Read the model definition and answer for the solid it produces. Units are mm, in the model's axes. A direction names the side the tool comes from. Round coordinates to 2 decimals unless told otherwise and drop trailing zeros. Write each loop counter-clockwise with the first axis right and the second up, starting at its lowest first coordinate (ties: lowest second). Pieces come first, ordered by that corner, then holes. Notation, with made-up numbers: (26.5, 6) - (48.5, 6) arc R14 ccw to (48.5, 24) - close; hole circle Ø3 at (83.25, 38). An arc over 180 degrees is marked (long way). One line per item, written item: value. Start each with the question number.
(1) A cutting plane is placed at B-B, the plane x = 0. Determine the outline of the cut face in (y, z).
(2) For faces 4 (the face through (39, 10.483, 9)), 5 (the face through (-1.172, 8.923, 17.902)), 6 (the face through (-39, 10.483, 9)), determine the directions among +Z, -Z, +X, -X, +Y, -Y from which every point of the face is accessible in a straight line to the end or side of a thin tool.
(3) The mould has two halves that part along Y. Classify faces 1 (the face through (12, 0, 11)), 2 (the face through (-25, 11, 15)), 3 (the face through (-56.5, 0.2, 5.4)): +Y half, -Y half, draft (parallel to the pull), parting line (faces both ways), or undercut.
(4) A cutting plane is placed at C-C, the plane y = 22. Determine the outline of the cut face in (x, z).
(5) A cutting plane is placed at A-A, the plane z = 4.5. Determine the outline of the cut face in (x, y).
(6) A cutting plane is placed at D-D, the plane x = -44.5. Determine the outline of the cut face in (y, z).
(7) Flat-ended cylindrical pins translate along their axes: pin 1 Ø17 at (x, y) = (42, 5) entering from +Z; pin 2 Ø4 at (y, z) = (-10.5, 15) entering from -X; pin 3 Ø8 at (x, y) = (-32.5, 15.5) entering from +Z; pin 4 Ø9 at (x, y) = (-45, 0) entering from +Z. Find the tip coordinate at first contact, or state that the pin passes through.
(8) Find the intervals of material crossed by L1, parallel to Y at x = 0, z = 13; L2, parallel to X at y = -4, z = 12.5; L3, parallel to Y at x = 0, z = 17, in increasing order.
from build123d import *

# Parameters (mm, degrees)
F0_R     = 5
F1_DEPTH = 11
F0_R_2   = 27
F2_DEPTH = 15
F0_R_3   = 9
F3_DEPTH = 11
F0_R_4   = 6
F4_DEPTH = 25
F5_DEPTH = 8


with BuildPart() as f1:
    # F0 (on Top) → F1 (new body)
    with BuildSketch(Plane.XY):
        with BuildLine():
            ThreePointArc((-28.108751, -10.48323), (-30, 0), (-28.108751, 10.48323))
            Line((-28.108751, 10.48323), (-49.727778, 10.48323))
            ThreePointArc((-49.727778, 10.48323), (-56.5, 0), (-49.727778, -10.48323))
            Line((-49.727778, -10.48323), (-28.108751, -10.48323))
        make_face()
        with Locations((-45, 0)):
            Circle(F0_R, mode=Mode.SUBTRACT)
        with BuildLine():
            ThreePointArc((28.108751, 10.48323), (29.523402, 5.326231), (30, 0))
            ThreePointArc((30, 0), (29.523402, -5.326231), (28.108751, -10.48323))
            Line((28.108751, -10.48323), (49.727778, -10.48323))
            ThreePointArc((49.727778, -10.48323), (56.5, 0), (49.727778, 10.48323))
            Line((49.727778, 10.48323), (28.108751, 10.48323))
        make_face()
        with Locations((45, 0)):
            Circle(F0_R, mode=Mode.SUBTRACT)
    extrude(amount=F1_DEPTH)

    # F0 (on Top) → F2 (join)
    with BuildSketch(Plane.XY):
        with BuildLine():
            ThreePointArc((28.108751, -10.48323), (29.523402, -5.326231), (30, 0))
            ThreePointArc((30, 0), (29.523402, 5.326231), (28.108751, 10.48323))
            ThreePointArc((28.108751, 10.48323), (21.908718, 20.494098), (12.333333, 27.347557))
            ThreePointArc((12.333333, 27.347557), (0, 30), (-12.333333, 27.347557))
            ThreePointArc((-12.333333, 27.347557), (-21.908718, 20.494098), (-28.108751, 10.48323))
            ThreePointArc((-28.108751, 10.48323), (-30, 0), (-28.108751, -10.48323))
            ThreePointArc((-28.108751, -10.48323), (-21.908718, -20.494098), (-12.333333, -27.347557))
            ThreePointArc((-12.333333, -27.347557), (0, -30), (12.333333, -27.347557))
            ThreePointArc((12.333333, -27.347557), (21.908718, -20.494098), (28.108751, -10.48323))
        make_face()
        Circle(F0_R_2, mode=Mode.SUBTRACT)
    extrude(amount=F2_DEPTH)

    # F0 (on Top) → F3 (join)
    with BuildSketch(Plane.XY):
        Circle(F0_R_2)
        Circle(F0_R_3, mode=Mode.SUBTRACT)
    extrude(amount=F3_DEPTH)

    # F0 (on Top) → F4 (join)
    with BuildSketch(Plane.XY):
        Circle(F0_R_3)
        Circle(F0_R_4, mode=Mode.SUBTRACT)
    extrude(amount=F4_DEPTH)

    # F0 (on Top) → F5 (join)
    with BuildSketch(Plane.XY):
        with BuildLine():
            Line((-49.727778, -10.48323), (-12.333333, -27.347557))
            ThreePointArc((-12.333333, -27.347557), (-21.908718, -20.494098), (-28.108751, -10.48323))
            Line((-28.108751, -10.48323), (-49.727778, -10.48323))
        make_face()
        with BuildLine():
            Line((49.727778, -10.48323), (28.108751, -10.48323))
            ThreePointArc((28.108751, -10.48323), (21.908718, -20.494098), (12.333333, -27.347557))
            Line((12.333333, -27.347557), (49.727778, -10.48323))
        make_face()
        with BuildLine():
            ThreePointArc((-28.108751, 10.48323), (-21.908718, 20.494098), (-12.333333, 27.347557))
            Line((-12.333333, 27.347557), (-49.727778, 10.48323))
            Line((-49.727778, 10.48323), (-28.108751, 10.48323))
        make_face()
        with BuildLine():
            ThreePointArc((12.333333, 27.347557), (21.908718, 20.494098), (28.108751, 10.48323))
            Line((28.108751, 10.48323), (49.727778, 10.48323))
            Line((49.727778, 10.48323), (12.333333, 27.347557))
        make_face()
    extrude(amount=F5_DEPTH)


solid = f1.part
Here are the results:
1. outline: (-30, 0) - (-6, 0) - (-6, 25) - (-9, 25) - (-9, 11) - (-27, 11) - (-27, 15) - (-30, 15) - close; (6, 0) - (30, 0) - (30, 15) - (27, 15) - (27, 11) - (9, 11) - (9, 25) - (6, 25) - close
2. face 4: +Z, +X, +Y
2. face 5: +Z
2. face 6: +Z, -X, +Y
3. face 1: undercut
3. face 2: draft
3. face 3: parting line
4. outline: (-24.19, 0) - (24.19, 0) - (24.19, 8) - (20.4, 8) - (20.4, 15) - (15.65, 15) - (15.65, 11) - (-15.65, 11) - (-15.65, 15) - (-20.4, 15) - (-20.4, 8) - (-24.19, 8) - close
5. outline: (-49.73, -10.48) - (-12.33, -27.35) arc R30 ccw to (12.33, -27.35) - (49.73, -10.48) arc R11.5 ccw to (49.73, 10.48) - (12.33, 27.35) arc R30 ccw to (-12.33, 27.35) - (-49.73, 10.48) arc R11.5 ccw to start; hole circle Ø10 at (-45, 0); hole circle Ø12 at (0, 0); hole circle Ø10 at (45, 0)
6. outline: (-12.84, 0) - (-4.97, 0) - (-4.97, 11) - (-10.48, 11) - (-10.48, 8) - (-12.84, 8) - close; (4.97, 0) - (12.84, 0) - (12.84, 8) - (10.48, 8) - (10.48, 11) - (4.97, 11) - close
7. pin 1: z = 11
7. pin 2: x = -28.77
7. pin 3: z = 8
7. pin 4: through
8. L1: -30 to -27, -9 to -6, 6 to 9, 27 to 30
8. L2: -29.73 to -26.7, -8.06 to -4.47, 4.47 to 8.06, 26.7 to 29.73
8. L3: -9 to -6, 6 to 9
